Could you check a few things on this model? Use its own coordinates, in mm. A direction names the side the tool comes from. Coordinates: 2 decimals unless noted, no trailing zeros. Order: outer loops, then holes, each group sorted by start corner. A loop starts at its lowest first (then second) coordinate and runs counter-clockwise, first axis right, second up. Notation, with made-up numbers: (27.25, -37) -> (86.25, -37) arc R35 cw to (86.25, 1) -> close; hole circle Ø5 at (-7.5, 10). An arc over 180 degrees is marked (long way). Use a Markdown table: item, result. Add a question column.
1) If I drill on L1, parallel to X at y = 9.25, z = -26.5; L2, parallel to Z at x = -22.5, y = 4.25; L3, parallel to X at y = -12.75, z = -22, over which ranges is the centre line in solid material (lowest first)? Write a range as [from, to].
2) If we section it at A-A (y = -4): Write out the boundary of the cut face in (x, z).
3) Which directions (+Z, -Z, +X, -X, +Y, -Y) give clear straight access to the entire face, cutting with the end or side of a thin tool? Please do faces 4 (the flat face through (163, 12, -30.287)), 5 (the flat face through (167.21, 12, -34)), 6 (the flat face through (130.186, 12, 4)).
4) If we section it at D-D (z = -47.5): Write out the boundary of the cut face in (x, y).
5) If we section it at C-C (x = 66.5): Write out the boundary of the cut face in (y, z).
6) Thinking about a two-plate mould opening in X: for faces 1 (the flat face through (-19.125, -7, -15)), 2 (the cylindrical face through (119.005, 5.07, -55.898)), 3 (the flat face through (163, 12, -37.803)), which applies, +X half, -X half, draft (parallel to the pull), parting line (faces both ways), or undercut?
7) Will these pins go through, and if not, where does the flat tip stop? pin 1 Ø4.5 at (y, z) = (-10.5, -22) entering from -X; pin 2 Ø4 at (x, y) = (164.5, 13) entering from +Z; pin 3 Ø2.5 at (x, y) = (164.5, 11.5) entering from -Z.
8) If we section it at B-B (z = -19.5): Write out the boundary of the cut face in (x, y), plus the area to 3 significant figures.
```python
from build123d import *

# Parameters (mm, degrees)
SKETCH2_W               = 300
SKETCH2_H               = 100
BOSS_EXTRUDE1_DEPTH     = 10
SKETCH3_W               = 32.480865485
SKETCH3_H               = 5
CUT_EXTRUDE4_DEPTH      = 100
FILLET2_R               = 10
FILLET3_R               = 10
SKETCH6_R               = 1.8
CUT_EXTRUDE11_DEPTH     = 100
SKETCH10_W              = 6.800425214
SKETCH10_H              = 7.704447869
SKETCH10_R              = 1.8
SKETCH10_W_2            = 7.232198243
SKETCH10_H_2            = 7.417822841
SKETCH10_W_3            = 7.704447868
SKETCH10_H_3            = 7.016311729
SKETCH10_W_4            = 7.663971273
SKETCH10_H_4            = 7.516208799
BOSS_EXTRUDE3_DEPTH     = 5
SKETCH11_R              = 5.007661082
CUT_EXTRUDE13_DEPTH     = 30
CROQUIS2_W              = 7.110286561
CROQUIS2_H              = 33
CROQUIS2_W_2            = 8.127928254
SALIENTE_EXTRUIR1_DEPTH = 15
SKETCH8_R               = 2.25
CORTAR_EXTRUIR1_DEPTH   = 50


with BuildPart() as part:
    # Sketch2 → Boss-Extrude1 (new body)
    with BuildSketch(Plane(origin=(0, 0, 0), x_dir=(1, 0, 0), z_dir=(0, 1, 0))):
        with Locations((30.996437266, 14.831990454)):
            Rectangle(SKETCH2_W, SKETCH2_H)
    extrude(amount=BOSS_EXTRUDE1_DEPTH)

    # Sketch3 → Cut-Extrude4 (cut)
    with BuildSketch(Plane.XY.offset(35.168009546)):
        with Locations((-102.763129992, 2.5)):
            Rectangle(SKETCH3_W, SKETCH3_H)
    extrude(amount=-CUT_EXTRUDE4_DEPTH, mode=Mode.SUBTRACT)

    # Fillet2
    fillet2_edges = [part.edges().sort_by_distance(p)[0] for p in [
        (180.996437266, 5, -64.831990454),
        (180.996437266, 5, 35.168009546),
    ]]
    fillet(fillet2_edges, radius=FILLET2_R)

    # Fillet3
    fillet3_edges = [part.edges().sort_by_distance(p)[0] for p in [
        (-119.003562734, 7.5, -64.831990454),
        (-119.003562734, 7.5, 35.168009546),
    ]]
    fillet(fillet3_edges, radius=FILLET3_R)

    # Sketch6 → Cut-Extrude11 (cut)
    with BuildSketch(Plane(origin=(0, 10, 0), x_dir=(1, 0, 0), z_dir=(0, 1, 0))):
        with Locations((125.905144225, 34.121382773)):
            Circle(SKETCH6_R)
        with Locations((126.546416062, -3.163994016)):
            Circle(SKETCH6_R)
        with Locations((163.282131276, -3.71365559)):
            Circle(SKETCH6_R)
        with Locations((163.465351801, 34.39621356)):
            Circle(SKETCH6_R)
    extrude(amount=-CUT_EXTRUDE11_DEPTH, mode=Mode.SUBTRACT)

    # Sketch10 → Boss-Extrude3 (add)
    with BuildSketch(Plane(origin=(0, 10, 0), x_dir=(1, 0, 0), z_dir=(0, 1, 0))):
        with Locations((125.922054042, 34.139208999)):
            Rectangle(SKETCH10_W, SKETCH10_H)
        with Locations((125.905144225, 34.121382773)):
            Circle(SKETCH10_R, mode=Mode.SUBTRACT)
        with Locations((126.569713587, -3.685857636)):
            Rectangle(SKETCH10_W_2, SKETCH10_H_2)
        with Locations((126.546416062, -3.163994016)):
            Circle(SKETCH10_R, mode=Mode.SUBTRACT)
        with Locations((163.380664231, -4.024818367)):
            Rectangle(SKETCH10_W_3, SKETCH10_H_3)
        with Locations((163.282131276, -3.71365559)):
            Circle(SKETCH10_R, mode=Mode.SUBTRACT)
        with Locations((163.378364349, 34.045089464)):
            Rectangle(SKETCH10_W_4, SKETCH10_H_4)
        with Locations((163.465351801, 34.39621356)):
            Circle(SKETCH10_R, mode=Mode.SUBTRACT)
    extrude(amount=BOSS_EXTRUDE3_DEPTH)

    # Sketch11 → Cut-Extrude13 (cut)
    with BuildSketch(Plane(origin=(0, 10, 0), x_dir=(1, 0, 0), z_dir=(0, 1, 0))):
        with Locations((114.379298218, 57.815546059)):
            Circle(SKETCH11_R)
        with Locations((113.986464963, -27.822103537)):
            Circle(SKETCH11_R)
    extrude(amount=-CUT_EXTRUDE13_DEPTH, mode=Mode.SUBTRACT)

    # Croquis2 → Saliente-Extruir1 (add)
    with BuildSketch(Plane.XZ):
        with Locations((-22.680335873, -14.831990454)):
            Rectangle(CROQUIS2_W, CROQUIS2_H)
        with Locations((-49.939598607, -14.831990454)):
            Rectangle(CROQUIS2_W_2, CROQUIS2_H)
    extrude(amount=SALIENTE_EXTRUIR1_DEPTH)

    # Sketch8 → Cortar-Extruir1 (cut)
    with BuildSketch(Plane(origin=(0, 10, 0), x_dir=(1, 0, 0), z_dir=(0, 1, 0))):
        with Locations((-49.690211369, 27.018639088)):
            Circle(SKETCH8_R)
        with Locations((-49.690211369, 2.645341819)):
            Circle(SKETCH8_R)
        with Locations((-22.549681442, 27.018639088)):
            Circle(SKETCH8_R)
        with Locations((-22.549681442, 2.645341819)):
            Circle(SKETCH8_R)
    extrude(amount=-CORTAR_EXTRUIR1_DEPTH, mode=Mode.SUBTRACT)


solid = part.part
```
Answer sheet:
| question | item | result |
|---|---|---|
| 1 | L1 | [-119, -51.88], [-47.5, -24.74], [-20.36, 181] |
| 1 | L2 | [-64.83, -29.27], [-24.77, -4.89], [-0.4, 35.17] |
| 1 | L3 | [-54, -45.88], [-26.24, -19.13] |
| 2 | outline | (-54, -31.33) -> (-45.88, -31.33) -> (-45.88, 1.67) -> (-54, 1.67) -> close; (-26.24, -31.33) -> (-19.13, -31.33) -> (-19.13, 1.67) -> (-26.24, 1.67) -> close; hole circle Ø4.5 at (-49.69, -27.02); hole circle Ø4.5 at (-49.69, -2.65); hole circle Ø4.5 at (-22.55, -27.02); hole circle Ø4.5 at (-22.55, -2.65) |
| 3 | face 4 | +X, -X, +Y |
| 3 | face 5 | +Z, -Z, +X, +Y |
| 3 | face 6 | +Z, -Z, +Y |
| 4 | outline | (-119, 5) -> (-86.52, 5) -> (-86.52, 0) -> (181, 0) -> (181, 10) -> (-119, 10) -> close |
| 5 | outline | (0, -64.83) -> (10, -64.83) -> (10, 35.17) -> (0, 35.17) -> close |
| 6 | face 1 | +X half |
| 6 | face 2 | undercut |
| 6 | face 3 | draft |
| 7 | pin 1 | x = -54 |
| 7 | pin 2 | z = 7.53 |
| 7 | pin 3 | z = -37.8 |
| 8 | outline | (-119, 5) -> (-86.52, 5) -> (-86.52, 0) -> (-54, 0) -> (-54, -15) -> (-45.88, -15) -> (-45.88, 0) -> (-26.24, 0) -> (-26.24, -15) -> (-19.13, -15) -> (-19.13, 0) -> (181, 0) -> (181, 10) -> (-119, 10) -> close |
| 8 | area | 3,070 mm2 |
